Work out the finished part from the listing and answer in its coordinate system (mm). A direction names the side the tool comes from. Give positions to 0.01 mm unless a question says otherwise; leave off trailing zeros. Order: outer loops, then holes, each group sorted by start corner. A loop starts at its lowest first (then second) coordinate and runs counter-clockwise, first axis right, second up. Notation, with made-up numbers: (-19.5, 3.5) - (8.5, 3.5) arc R6 ccw to (8.5, 11.5) - close; hole circle Ø4 at (80.25, -19.75). An arc over 180 degrees is marked (long way). Put each result on its own line as item: value.
Autodesk Inventor part; units mm, degrees
ref_plane "YZ Plane" through (0, 0, 0) normal (1, 0, 0) x (0, 1, 0)
ref_plane "XZ Plane" through (0, 0, 0) normal (0, 1, 0) x (-1, 0, 0)
ref_plane "XY Plane" through (0, 0, 0) normal (0, 0, 1) x (1, 0, 0)
sketch "Skizze1" plane through (0, 0, 0) normal (0, 0, 1) x (1, 0, 0)
  line L0 (0, 0) -> (20.5, 0) construction
  circle A0 centre (-25, 0) radius 2.25 construction
  line L1 (-25, 0) -> (0, 0) construction
  line L2 (-26, -9.9499) -> (-1.25, -12.4373)
  line L3 (-1.25, 12.4373) -> (-26, 9.9499)
  arc A1 (-26, 9.9499) -> (-26, -9.9499) centre (-25, 0) ccw
  arc A2 (-1.25, -12.4373) -> (-1.25, 12.4373) centre (0, 0) ccw construction
  circle A3 centre (0, 0) radius 4
  arc A4 (8.6207, 9.0517) -> (12.5, 7.5) centre (12.5, 13.125) ccw
  arc A5 (12.5, -7.5) -> (8.6207, -9.0517) centre (12.5, -13.125) ccw
  line L4 (12.5, 7.5) -> (20.5, 7.5)
  line L5 (20.5, 7.5) -> (20.5, -7.5)
  line L6 (20.5, -7.5) -> (12.5, -7.5)
  line L7 (12.5, -7.5) -> (12.5, 7.5) construction
  arc A6 (-1.25, -12.4373) -> (8.6207, -9.0517) centre (0, 0) ccw
  arc A7 (8.6207, 9.0517) -> (-1.25, 12.4373) centre (0, 0) ccw
  circle A8 centre (-25, 0) radius 4.875 construction
  line L8 (-25, 0) -> (-25, 4.875) construction
  circle A9 centre (0, 0) radius 10.15 construction
  line L9 (0, 0) -> (0, -10.15) construction
  line L10 (16.5, 5.25) -> (16.5, -5.25) construction
  line L11 (16.5, 7.5) -> (16.5, -7.5) construction
  circle A10 centre (-25, 0) radius 10 construction
  line L12 (-25, 0) -> (-13.7735, -8.3646) construction
  line L13 (-13.7735, -8.3646) -> (-14.0535, -11.1505) construction
  line L14 (-25, 0) -> (-13.7735, 8.3646) construction
  line L15 (-13.7735, 8.3646) -> (-14.0535, 11.1505) construction
  point P0 (-12.5, 0)
  point P1 (12.5, 0)
  point P2 (-29.2219, -2.4375)
  point P3 (-20.7781, -2.4375)
  point P4 (0, -10.15)
  point P5 (0, 10.15)
  point P6 (16.5, 0)
  dimension "d127" = 20.3
  dimension "Flansch_Hole_Dia" = 9.75
  dimension "d101" = 0
  dimension "CounterWeight_Swing_Rad" = 25
  dimension "d103" = 4.5
  dimension "d105" = 8
  dimension "d106" = 15
  dimension "LowerArm_ShaftFixation_Width" = 8
  dimension "d118" = 360
  dimension "d130" = 360
  dimension "d132" = 10.5
  dimension "d140" = 12.5
  dimension "LowerArm_Back_DiaOut" = 20
  dimension "d142" = 2.8
  dimension "LowerArm_Cover_FixationHole" = 14
  dimension "d144" = 14
  dimension "d145" = 2.8
extrude "Grundprofil" add sketch "Skizze1" along normal blind 2
hole "Hole10" at (-13.7735, -8.3646, 0) at (-13.7735, 8.3646, 0) direction (0, 0, 1) diameter 2.2 depth 12 tip angle 118 countersink diameter 4.4 countersink angle 90
hole "Hole11" at (16.5, 5.25, 0) at (16.5, -5.25, 0) direction (0, 0, 1) diameter 2.2 depth 3 tip angle 118 countersink diameter 4.4 countersink angle 90
hole "Hole12" at (-25, 0, 0) direction (0, 0, 1) diameter 3.2 depth 12 tip angle 118 countersink diameter 6.3 countersink angle 90
properties part number "Lower_Arm_v3" material "Aluminum 6061"
(1) Section D-D, the plane z = 0.8 is taken. Write down the section's boundary in (x, y), then the cut area to 3 significant figures.
Geometry check:
outline: (-26, -9.95) - (-1.25, -12.44) arc R12.5 ccw to (8.62, -9.05) arc R5.63 cw to (12.5, -7.5) - (20.5, -7.5) - (20.5, 7.5) - (12.5, 7.5) arc R5.62 cw to (8.62, 9.05) arc R12.5 ccw to (-1.25, 12.44) - (-26, 9.95) arc R10 ccw to start; hole circle Ø4.7 at (-25, 0); hole circle Ø2.8 at (-13.77, -8.36); hole circle Ø2.8 at (-13.77, 8.36); hole circle Ø8 at (0, 0); hole circle Ø2.8 at (16.5, -5.25); hole circle Ø2.8 at (16.5, 5.25)
area: 1,010 mm²
(2) Straight lines are drawn through the part: line 1 (Y direction, x = 16, z = 1); line 2 (X direction, y = 4.75, z = 0.4); line 3 (X direction, y = 1, z = 0.9). For each, find the intervals that lie inside material, in ascending order.
Geometry check:
line 1: y = -7.5 to -6.34, -4.16 to 4.16, 6.34 to 7.5
line 2: x = -33.8 to 14.77, 18.23 to 20.5
line 3: x = -34.95 to -27.02, -22.98 to -3.87, 3.87 to 20.5
(3) A tool of negligible diameter and unlimited length cuts with its end or side. For faces 4 (the face through (-13.798, -11.176, 0.986)), 5 (the face through (16, 7.5, 1)), from which of +Z, -Z, +X, -X, +Y, -Y can it reach the whole face along a straight path? Write none if from no direction.
Geometry check:
face 4: +Z, -Z, -X, -Y
face 5: +Z, -Z, +X, +Y
(4) Determine the mould class of faces 1 (the face through (20.5, 0, 1)), 2 (the face through (-24.03, -1.27, 1.78)), 3 (the face through (-13.45, 11.21, 0.99)) for opening direction X: pulls with the +X half, pulls with the -X half, needs draft (parallel to the pull), parting line crosses it, or undercut.
Geometry check:
face 1: pulls with the +X half
face 2: undercut
face 3: pulls with the -X half
(5) Section B-B, the plane x = 0 is taken. Write down the section's boundary in (y, z), then the cut area to 3 significant figures.
Geometry check:
outline: (-12.5, 0) - (-4, 0) - (-4, 2) - (-12.5, 2) - close; (4, 0) - (12.5, 0) - (12.5, 2) - (4, 2) - close
area: 34.0 mm²
(6) Given pin 1 (2 mm diameter, centred on x = 16.5, y = 5.25, fed in from +Z); pin 2 (2.5 mm diameter, centred on x = 16.5, y = -5.25, fed in from -Z); pin 3 (1 mm diameter, centred on x = 18, z = 1, fed in from +Y); pin 4 (3.5 mm diameter, centred on x = -25, y = 0, fed in from -Z), each flat-ended and moving along its own axis, determine where each tip first touches the part or whether it passes through.
Geometry check:
pin 1: passes through
pin 2: stops at z = 0.95
pin 3: stops at y = 7.5
pin 4: stops at z = 1.4
(7) Section C-C, the plane y = 0 is taken. Write down the section's boundary in (x, z), then the cut area to 3 significant figures.
Geometry check:
outline: (-35, 0) - (-28.15, 0) - (-26.6, 1.55) - (-26.6, 2) - (-35, 2) - close; (-23.4, 1.55) - (-21.85, 0) - (-4, 0) - (-4, 2) - (-23.4, 2) - close; (4, 0) - (20.5, 0) - (20.5, 2) - (4, 2) - close
area: 86.2 mm²
(8) Section A-A, the plane x = 16.5 is taken. Write down the section's boundary in (y, z), then the cut area to 3 significant figures.
Geometry check:
outline: (-7.5, 0) - (-7.45, 0) - (-6.35, 1.1) - (-6.35, 2) - (-7.5, 2) - close; (-4.15, 1.1) - (-3.05, 0) - (3.05, 0) - (4.15, 1.1) - (4.15, 2) - (-4.15, 2) - close; (6.35, 1.1) - (7.45, 0) - (7.5, 0) - (7.5, 2) - (6.35, 2) - close
area: 18.8 mm²
